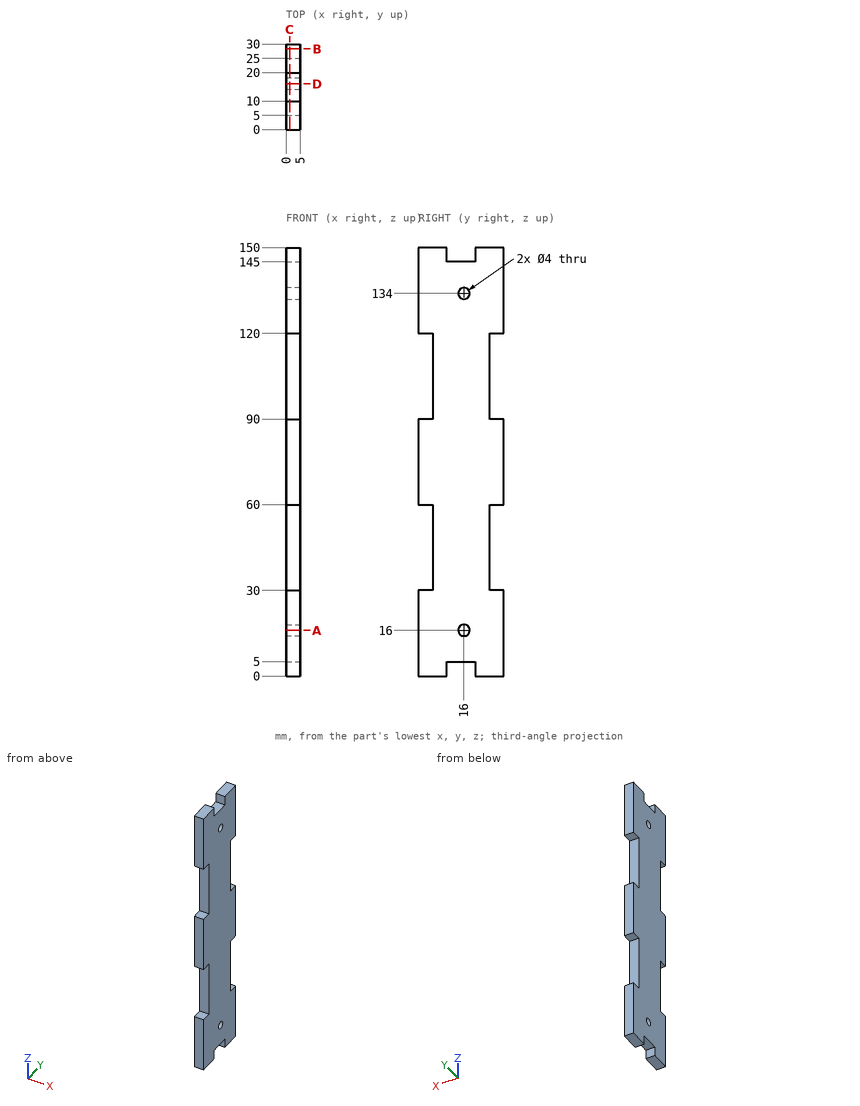
Could you check a few things on this drawing? It's one solid part, dimensions in mm from its lowest x, y, z. Coordinates: 2 decimals unless noted, no trailing zeros. Order: outer loops, then holes, each group sorted by start corner. A loop starts at its lowest first (then second) coordinate and runs counter-clockwise, first axis right, second up. Notation, with made-up numbers: (81, 8) - (116, 8) arc R16 ccw to (116, 26) - close; hole circle Ø8 at (-6, 52.5). An arc over 180 degrees is marked (long way). Answer as a JSON object with one key per item and string values. Group by question number.
Q1. Imagine slicing it at D-D (y = 16). Please give me the cut outline in (x, z).
Q2. Will these pins go through, and if not, where does the flat tip stop? P1, Ø3, axis at x = 1.5, z = 45.5, coming from the -Y side; P2, Ø2.5, axis at x = 2.5, y = 16, coming from the +Z side; P3, Ø1.5, axis at x = 3.5, y = 13.5, coming from the -Z side.
Q3. I need wall thicknesses on line 1 (Z direction, x = 0.5, y = 4.25); line 2 (Z direction, x = 1.65, y = 15.25); line 3 (Y direction, x = 3.7, z = 134). Which ranges of each line are inside material? Lowest first, please. Write a range as from..to.
Q4. Imagine slicing it at A-A (z = 16). Please give me the cut outline in (x, y).
Q5. Imagine slicing it at C-C (x = 1.25). Give the number of separate pieces and of enclosed holes in the cut face, and give its area (3 significant figures).
Q6. Imagine slicing it at B-B (y = 28.25). Please give me the cut outline in (x, z).
Determined:
{
 "1": {"outline": "(0, 5) - (5, 5) - (5, 14) - (0, 14) - close; (0, 18) - (5, 18) - (5, 132) - (0, 132) - close; (0, 136) - (5, 136) - (5, 145) - (0, 145) - close"},
 "2": {"P1": "stops at y = 5", "P2": "stops at z = 145", "P3": "stops at z = 5"},
 "3": {"line 1": "z = 0..30, 60..90, 120..150", "line 2": "z = 5..14.15, 17.85..132.15, 135.85..145", "line 3": "y = 0..14, 18..30"},
 "4": {"outline": "(0, 0) - (5, 0) - (5, 14) - (0, 14) - close; (0, 18) - (5, 18) - (5, 30) - (0, 30) - close"},
 "5": {"separate pieces": "1", "enclosed holes": "2", "area": "3,770 mm2"},
 "6": {"outline": "(0, 0) - (5, 0) - (5, 30) - (0, 30) - close; (0, 60) - (5, 60) - (5, 90) - (0, 90) - close; (0, 120) - (5, 120) - (5, 150) - (0, 150) - close"}
}
